Autodesk Inventor part; units mm, degrees
ref_plane "YZ Plane" through (0, 0, 0) normal (1, 0, 0) x (0, 1, 0)
ref_plane "XZ Plane" through (0, 0, 0) normal (0, 1, 0) x (-1, 0, 0)
ref_plane "XY Plane" through (0, 0, 0) normal (0, 0, 1) x (1, 0, 0)
sketch "Sketch1" plane through (0, 0, 0) normal (0, 1, 0) x (-1, 0, 0)
  line L0 (9.98, 17.98) -> (-9.98, 17.98)
  line L1 (-9.98, 17.98) -> (-9.98, -17.98)
  line L2 (-9.98, -17.98) -> (9.98, -17.98)
  line L3 (9.98, -17.98) -> (9.98, 17.98)
  line L4 (9.98, 17.98) -> (-9.98, -17.98) construction
  line L5 (-9.98, 17.98) -> (9.98, -17.98) construction
  point P0 (0, 0)
  dimension "d0" = 35.96
  dimension "d1" = 19.96
extrude "arm-wall" add sketch "Sketch1" along normal blind 3
sketch "Sketch2" plane through (0, 3, 0) normal (0, 1, 0) x (1, 0, 0)
  line L0 (-8, -17.98) -> (8, -17.98)
  line L1 (8, -17.98) -> (8, 15.98)
  line L2 (8, 15.98) -> (-8, 15.98)
  line L3 (-8, 15.98) -> (-8, -17.98)
  line L4 (-8, -17.98) -> (8, 15.98) construction
  line L5 (8, -17.98) -> (-8, 15.98) construction
  line L6 (0, 25.172) -> (0, -25.172)
  line L7 (9.98, 17.98) -> (-9.98, 17.98)
  line L8 (-9.98, -17.98) -> (9.98, -17.98)
  point P0 (0, 0)
  point P1 (0, -1)
  point P2 (0, -1)
  dimension "d4" = 16
  dimension "d5" = 2
extrude "slot" cut sketch "Sketch2" against normal blind 2
fillet "Fillet1" radius 2 1 edges at (-9.98, 1.5, 17.98)
fillet "Fillet2" radius 2 1 edges at (9.98, 1.5, 17.98)
fillet "Fillet3" radius 2 1 edges at (9.98, 1.5, -17.98)
fillet "Fillet4" radius 2 1 edges at (-9.98, 1.5, -17.98)
equation "\"d2\" = armthick"
equation "\"d4\" = adapterh"
equation "\"d5\" = -0.5 * adapterw + 0.5 * armw"
equation "\"d6\" = armslotd"
equation "\"d8\" = cornerrad"
equation "\"d9\" = cornerrad"
equation "\"d10\" = cornerrad"
equation "\"d11\" = cornerrad"
equation "\"printer3dtolerance\" = 0.12"
equation "\"wallw\" = 42"
equation "\"wallh\" = 44"
equation "\"cornerrad\" = 2"
equation "\"baseextra\" = 2"
equation "\"wall1_thick\" = 8"
equation "\"wall2_thick\" = 6.4"
equation "\"wall3_thick\" = 4"
equation "\"wall1slot\" = 8.12"
equation "\"wall2slot\" = 6.52"
equation "\"wall3slot\" = 4.12"
equation "\"gap2\" = 28"
equation "\"baseh\" = 79.12"
equation "\"basew\" = 44"
equation "\"base_thick\" = 6"
equation "\"base_slots_depth\" = 4"
equation "\"servobigcircledia\" = 11.62"
equation "\"servosmallcircledia\" = 5.92"
equation "\"servo9gw\" = 22.8"
equation "\"servomounth\" = 4"
equation "\"servomountsquare\" = 6"
equation "\"servopolygonr\" = 6.12"
equation "\"servopolygonl\" = 5.92"
equation "\"distancefrombottom\" = 34"
equation "\"distancefromleft\" = 26"
equation "\"wall3slotd\" = 2"
equation "\"wall3slotw\" = 36"
equation "\"adapterh\" = 16"
equation "\"adapterw\" = 32"
equation "\"armw\" = 36"
equation "\"armslotd\" = 2"
equation "\"armthick\" = 3"
properties part number "adapter-slot"
Geometry check sheet. Reference: the model listing, model coordinates, mm. A direction names the side the tool comes from. Coordinates: 2 decimals unless noted, no trailing zeros. Loops run counter-clockwise (first coordinate to the right, second up) from the corner with the lowest first, then second, coordinate; pieces in that order, holes last.
Item 1: Sectioned sample at B-B, the plane y = 2.55. Record the boundary of the cut face in (x, z), then the cut area to 3 significant figures.
Item 2: Access from +Z, -Z, +X, -X, +Y, -Y to the whole of each face (thin tool, end or side, straight path). Record for faces 1 (the face through (-9.38, 1.52, -17.41)), 2 (the face through (0, 1, 1)).
Item 3: Sectioned sample at C-C, the plane x = -1.25. Record the boundary of the cut face in (y, z), then the cut area to 3 significant figures.
Item 4: Thickness scan on line 1 (X direction, y = 2.75, z = 8); line 2 (Y direction, x = 3, z = 3.5); line 3 (Z direction, x = 7.75, y = 2.15). Record the ranges inside material, lowest first.
Item 5: Sectioned sample at A-A, the plane z = 1. Record the boundary of the cut face in (x, y), then the cut area to 3 significant figures.
Item 6: Release check for a two-part mould opening along X. For faces 3 (the face through (8.2, 3, -1.2)), 4 (the face through (-9.98, 1, 0)), 5 (the face through (0, 2, -15.98)) record: released by +X, released by -X, zero draft, split by the parting line, or undercut.
Item 7: Go/stop test with flat-tipped pins: pin 1 Ø1.5 at (x, z) = (-3, -0.5) entering from +Y; pin 2 Ø0.6 at (x, y) = (2.5, 2.5) entering from +Z. Record where each tip stops, or that it passes through.
Check result:
1. outline: (-9.98, -15.98) arc R2 ccw to (-7.98, -17.98) - (7.98, -17.98) arc R2 ccw to (9.98, -15.98) - (9.98, 15.98) arc R2 ccw to (8, 17.98) - (8, -15.98) - (-8, -15.98) - (-8, 17.98) arc R2 ccw to (-9.98, 15.98) - close
1. area: 171 mm2
2. face 1: -Z, -X, +Y, -Y
2. face 2: +Z, +Y
3. outline: (0, -17.98) - (3, -17.98) - (3, -15.98) - (1, -15.98) - (1, 17.98) - (0, 17.98) - close
3. area: 40.0 mm2
4. line 1: x = -9.98 to -8, 8 to 9.98
4. line 2: y = 0 to 1
4. line 3: z = -17.98 to -15.98
5. outline: (-9.98, 0) - (9.98, 0) - (9.98, 3) - (8, 3) - (8, 1) - (-8, 1) - (-8, 3) - (-9.98, 3) - close
5. area: 27.9 mm2
6. face 3: zero draft
6. face 4: released by -X
6. face 5: undercut
7. pin 1: stops at y = 1
7. pin 2: stops at z = -15.98
